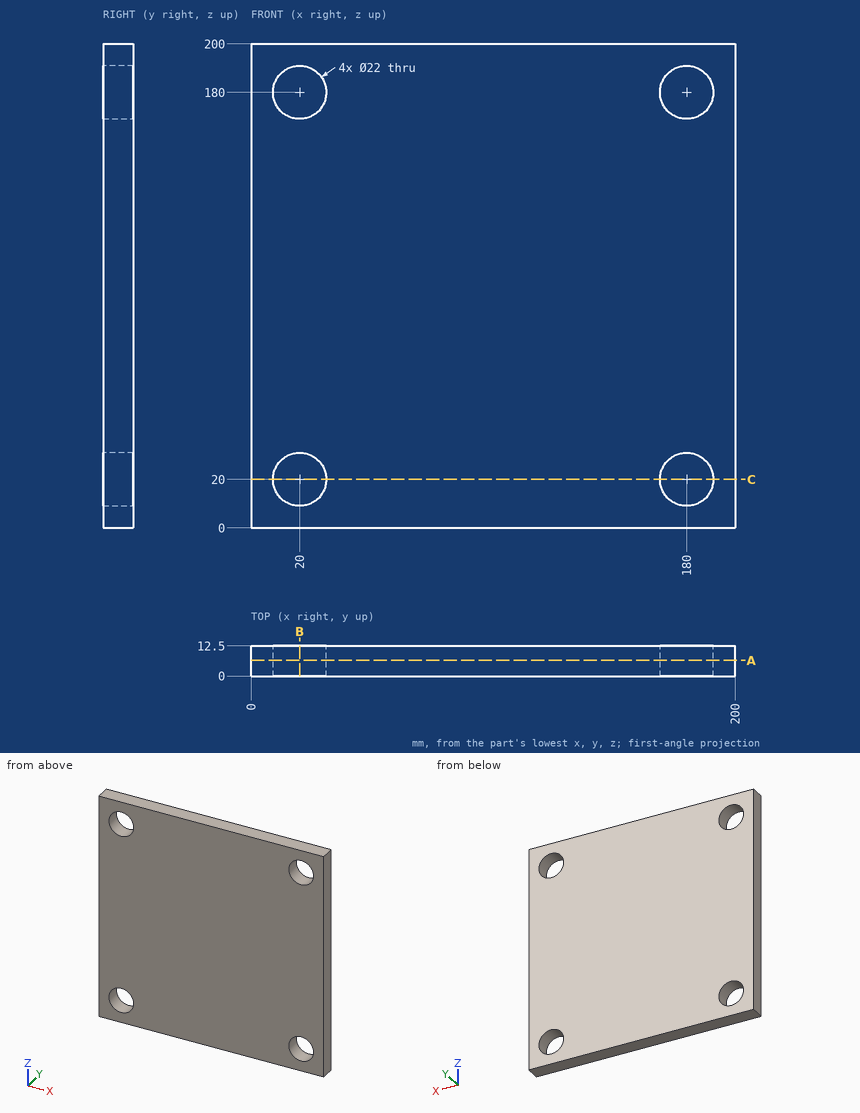
Answer from the drawing. Dimensions are ordinates in mm from the lowest x, y and z of the part. Round coordinates to 2 decimals unless told otherwise and drop trailing zeros. Order: outer loops, then holes, each group sorted by start corner. A loop starts at its lowest first (then second) coordinate and runs counter-clockwise, first axis right, second up. Notation, with made-up numbers: (63.25, 70.5) - (114.25, 70.5) arc R19 cw to (114.25, 98.5) - close; hole circle Ø5 at (78.5, 15.25). An arc over 180 degrees is marked (long way). Put each result on its own line as item: value. Start each with the question number.
(1) Find section B-B (x = 20). Give the vertices of the cut face in (y, z).
(2) Find section C-C (z = 20). Give the vertices of the cut face in (x, y), plus the area to 3 significant figures.
(3) Straight lines are drawn through the part: probe 1 along X at (y, z) = (6.5, 20); probe 2 along Z at (x, y) = (170, 6.25); probe 3 along Z at (x, y) = (23.5, 4). For each, find the intervals that lie inside material, in ascending order. Write a range as from..to.
(4) Find section A-A (y = 6.5). Give the vertices of the cut face in (x, z).
(5) Given P1, Ø2, axis at x = 22, y = 9, coming from the -Z side; P2, Ø17.5, axis at x = 20, z = 20, coming from the -Y side, each flat-ended and moving along its own axis, determine where each tip first touches the part or whether it passes through.
Reply:
1. outline: (0, 0) - (12.5, 0) - (12.5, 9) - (0, 9) - close; (0, 31) - (12.5, 31) - (12.5, 169) - (0, 169) - close; (0, 191) - (12.5, 191) - (12.5, 200) - (0, 200) - close
2. outline: (0, 0) - (9, 0) - (9, 12.5) - (0, 12.5) - close; (31, 0) - (169, 0) - (169, 12.5) - (31, 12.5) - close; (191, 0) - (200, 0) - (200, 12.5) - (191, 12.5) - close
2. area: 1,950 mm^2
3. probe 1: 0..9, 31..169, 191..200
3. probe 2: 0..15.42, 24.58..175.42, 184.58..200
3. probe 3: 0..9.57, 30.43..169.57, 190.43..200
4. outline: (0, 0) - (200, 0) - (200, 200) - (0, 200) - close; hole circle Ø22 at (20, 20); hole circle Ø22 at (20, 180); hole circle Ø22 at (180, 20); hole circle Ø22 at (180, 180)
5. P1: z = 0
5. P2: through
